```python
from build123d import *

# Parameters (mm, degrees)
ESBO_O1_W                = 85.6
ESBO_O1_H                = 56
RESSALTO_EXTRUS_O1_DEPTH = 1.6
ESBO_O2_R                = 0.5
CORTE_EXTRUS_O1_DEPTH    = 2
ESBO_O3_R                = 1.25
CORTE_EXTRUS_O2_DEPTH    = 10


with BuildPart() as part:
    # Esboço1 → Ressalto-extrusão1 (new body)
    with BuildSketch(Plane(origin=(0, 0, 0), x_dir=(-1, 0, 0), z_dir=(0, 0, -1))):
        with Locations((0.3, 0)):
            Rectangle(ESBO_O1_W, ESBO_O1_H)
    extrude(amount=-RESSALTO_EXTRUS_O1_DEPTH)

    # Esboço2 → Corte-extrusão1 (cut)
    with BuildSketch(Plane.XY.offset(1.6)):
        with Locations((37, 6.6)):
            Circle(ESBO_O2_R)
        with Locations((34.3, 6.6)):
            Circle(ESBO_O2_R)
        with Locations((34.3, 4.05)):
            Circle(ESBO_O2_R)
        with Locations((34.3, 2.04)):
            Circle(ESBO_O2_R)
        with Locations((34.3, -0.4)):
            Circle(ESBO_O2_R)
        with Locations((37, 4.05)):
            Circle(ESBO_O2_R)
        with Locations((37, 2.04)):
            Circle(ESBO_O2_R)
        with Locations((37, -0.4)):
            Circle(ESBO_O2_R)
    extrude(amount=-CORTE_EXTRUS_O1_DEPTH, mode=Mode.SUBTRACT)

    # Esboço3 → Corte-extrusão2 (cut)
    with BuildSketch(Plane.XY.offset(1.6)):
        with Locations((37.6, 15.4)):
            Circle(ESBO_O3_R)
        with Locations((-17.6, -10)):
            Circle(ESBO_O3_R)
    extrude(amount=-CORTE_EXTRUS_O2_DEPTH, mode=Mode.SUBTRACT)


solid = part.part
```
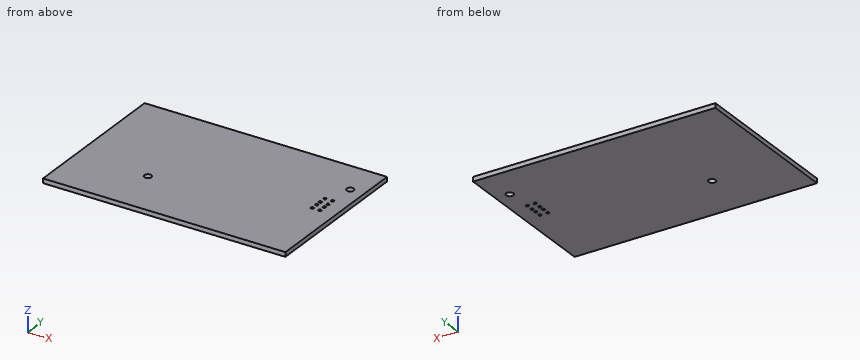
Geometry: final body of the model. Coordinates: model frame, mm. Give positions to 0.01 mm unless a question says otherwise; leave off trailing zeros. Loops run counter-clockwise (first coordinate to the right, second up) from the corner with the lowest first, then second, coordinate; pieces in that order, holes last. Notation, with made-up numbers: (66.25, 53.5) -> (103.25, 53.5) arc R24 ccw to (103.25, 80.5) -> close; hole circle Ø4 at (-1, 80.5). An arc over 180 degrees is marked (long way). Use CSV: the item, a comma, the result in double quotes.
(1) Ray query, line 1 along Y through (x, z) = (34.3, 0.45); line 2 along Y through (x, z) = (-17.6, 0.4). Return the intervals inside material, ascending. Write a range as [from, to].
From the geometry:
line 1,"[-28, -0.9], [0.1, 1.54], [2.54, 3.55], [4.55, 6.1], [7.1, 28]"
line 2,"[-28, -11.25], [-8.75, 28]"
(2) Cut plane B-B (x = -17.6). Output: boundary loops of the cut face in (y, z), plus the area to 3 significant figures.
From the geometry:
outline,"(-28, 0) -> (-11.25, 0) -> (-11.25, 1.6) -> (-28, 1.6) -> close; (-8.75, 0) -> (28, 0) -> (28, 1.6) -> (-8.75, 1.6) -> close"
area,"85.6 mm^2"
(3) First-contact query: P1, Ø4, axis at x = -17.6, y = -10, coming from the +Z side. Flat tip, straight axial feed; report the tip coordinate or a pass-through.
From the geometry:
P1,"z = 1.6"
(4) Cut plane A-A (y = -10). Output: boundary loops of the cut face in (x, z), plus the area to 3 significant figures.
From the geometry:
outline,"(-43.1, 0) -> (-18.85, 0) -> (-18.85, 1.6) -> (-43.1, 1.6) -> close; (-16.35, 0) -> (42.5, 0) -> (42.5, 1.6) -> (-16.35, 1.6) -> close"
area,"133 mm^2"
